from build123d import *

# Parameters (mm, degrees)
BOSS_EXTRUDE1_DEPTH      = 3
BOSS_EXTRUDE1_DEPTH_BACK = 4.55
SKETCH1_W                = 12
SKETCH1_H                = 10
SKETCH1_R                = 2.3
SKETCH1_H_2              = 28.075
SKETCH1_W_2              = 46.7
SKETCH5_W                = 12
SKETCH5_H                = 25.875
SKETCH5_H_2              = 10
SKETCH5_H_3              = 25.866
SKETCH5_W_2              = 46.7
CUT_EXTRUDE1_DEPTH       = 4.55
CUT_EXTRUDE2_DEPTH       = 87.014737759
CHAMFER1_SIZE            = 2
FILLET1_R                = 3
FILLET2_R                = 3


with BuildPart() as part:
    # Sketch1 → Boss-Extrude1 (new, two sides: drawn at the far end of the back side and taken through both)
    # profile 1 of 11: a face of its own
    with BuildSketch(Plane.XY.offset(-BOSS_EXTRUDE1_DEPTH_BACK)):
        with Locations((-38.872559152, 32.371494367)):
            Rectangle(SKETCH1_W, SKETCH1_H)
        with Locations((-38.872559152, 32.371494367)):
            Circle(SKETCH1_R, mode=Mode.SUBTRACT)
    # profile 2 of 11: a face of its own
    with BuildSketch(Plane.XY.offset(-BOSS_EXTRUDE1_DEPTH_BACK)):
        with Locations((-38.872559152, 13.333994367)):
            Rectangle(SKETCH1_W, SKETCH1_H_2)
    # profile 3 of 11: a face of its own
    with BuildSketch(Plane.XY.offset(-BOSS_EXTRUDE1_DEPTH_BACK)):
        with Locations((-38.872559152, -5.703505633)):
            Rectangle(SKETCH1_W, SKETCH1_H)
    # profile 4 of 11: a face of its own
    with BuildSketch(Plane.XY.offset(-BOSS_EXTRUDE1_DEPTH_BACK)):
        with Locations((-38.872559152, -24.741005633)):
            Rectangle(SKETCH1_W, SKETCH1_H_2)
    # profile 5 of 11: a face of its own
    with BuildSketch(Plane.XY.offset(-BOSS_EXTRUDE1_DEPTH_BACK)):
        with Locations((-38.872559152, -43.778505633)):
            Rectangle(SKETCH1_W, SKETCH1_H)
        with Locations((-38.872559152, -43.778505633)):
            Circle(SKETCH1_R, mode=Mode.SUBTRACT)
    # profile 6 of 11: a face of its own
    with BuildSketch(Plane.XY.offset(-BOSS_EXTRUDE1_DEPTH_BACK)):
        with Locations((19.827440848, -24.741005633)):
            Rectangle(SKETCH1_W, SKETCH1_H_2)
    # profile 7 of 11: a face of its own
    with BuildSketch(Plane.XY.offset(-BOSS_EXTRUDE1_DEPTH_BACK)):
        with Locations((19.827440848, -43.778505633)):
            Rectangle(SKETCH1_W, SKETCH1_H)
        with Locations((19.827440848, -43.778505633)):
            Circle(SKETCH1_R, mode=Mode.SUBTRACT)
    # profile 8 of 11: a face of its own
    with BuildSketch(Plane.XY.offset(-BOSS_EXTRUDE1_DEPTH_BACK)):
        with Locations((19.827440848, -5.703505633)):
            Rectangle(SKETCH1_W, SKETCH1_H)
    # profile 9 of 11: a face of its own
    with BuildSketch(Plane.XY.offset(-BOSS_EXTRUDE1_DEPTH_BACK)):
        with Locations((-9.522559152, -5.703505633)):
            Rectangle(SKETCH1_W_2, SKETCH1_H)
    # profile 10 of 11: a face of its own
    with BuildSketch(Plane.XY.offset(-BOSS_EXTRUDE1_DEPTH_BACK)):
        with Locations((19.827440848, 13.333994367)):
            Rectangle(SKETCH1_W, SKETCH1_H_2)
    # profile 11 of 11: a face of its own
    with BuildSketch(Plane.XY.offset(-BOSS_EXTRUDE1_DEPTH_BACK)):
        with Locations((19.827440848, 32.371494367)):
            Rectangle(SKETCH1_W, SKETCH1_H)
        with Locations((19.827440848, 32.371494367)):
            Circle(SKETCH1_R, mode=Mode.SUBTRACT)
    extrude(amount=BOSS_EXTRUDE1_DEPTH + BOSS_EXTRUDE1_DEPTH_BACK)

    # Sketch5 → Cut-Extrude1 (cut)
    with BuildSketch(Plane(origin=(0, 0, -4.55), x_dir=(-1, 0, 0), z_dir=(0, 0, -1))):
        with Locations((-19.827440848, 12.233994367)):
            Rectangle(SKETCH5_W, SKETCH5_H)
        with Locations((-19.827440848, -5.703505633)):
            Rectangle(SKETCH5_W, SKETCH5_H_2)
        with Locations((-19.827440848, -23.636505633)):
            Rectangle(SKETCH5_W, SKETCH5_H_3)
        with Locations((9.522559152, -5.703505633)):
            Rectangle(SKETCH5_W_2, SKETCH5_H_2)
        with Locations((38.872559152, -5.703505633)):
            Rectangle(SKETCH5_W, SKETCH5_H_2)
        with Locations((38.872559152, -23.636505633)):
            Rectangle(SKETCH5_W, SKETCH5_H_3)
        with Locations((38.872559152, 12.233994367)):
            Rectangle(SKETCH5_W, SKETCH5_H)
    extrude(amount=-CUT_EXTRUDE1_DEPTH, mode=Mode.SUBTRACT)

    # Sketch6 → Cut-Extrude2 (cut, through all)
    with BuildSketch(Plane.ZY.offset(44.872559152)):
        Polygon((-1.05, 28.569847873), (3, 25.171494367), (3, 37.371494367), (-1.05, 37.371494367), align=None)
        Polygon((-1.05, -48.778505633), (3, -48.778505633), (3, -36.578505633), (-1.05, -39.976859139), align=None)
    extrude(amount=-CUT_EXTRUDE2_DEPTH, mode=Mode.SUBTRACT)

    # Chamfer1
    chamfer1_edges = [part.edges().sort_by_distance(p)[0] for p in [
        (-32.872559152, -10.703505633, 1.5),
        (13.827440848, -10.703505633, 1.5),
        (13.827440848, -0.703505633, 1.5),
        (-32.872559152, -0.703505633, 1.5),
    ]]
    chamfer(chamfer1_edges, length=CHAMFER1_SIZE)

    # Fillet1
    fillet1_edges = [part.edges().sort_by_distance(p)[0] for p in [
        (13.827440848, 37.371494367, -2.8),
        (25.827440848, 37.371494367, -2.8),
        (25.827440848, -48.778505633, -2.8),
        (13.827440848, -48.778505633, -2.8),
        (-32.872559152, -48.778505633, -2.8),
        (-44.872559152, -48.778505633, -2.8),
        (-44.872559152, 37.371494367, -2.8),
        (-32.872559152, 37.371494367, -2.8),
    ]]
    fillet(fillet1_edges, radius=FILLET1_R)

    # Fillet2
    fillet2_edges = [part.edges().sort_by_distance(p)[0] for p in [
        (-38.872559152, -36.578505633, 3),
        (-38.872559152, 25.171494367, 3),
        (19.827440848, 25.171494367, 3),
        (19.827440848, -36.578505633, 3),
    ]]
    fillet(fillet2_edges, radius=FILLET2_R)


solid = part.part
Input: part model. Units: mm. Frame: model coordinates. A direction names the side the tool comes from. Give positions to 0.01 mm unless a question says otherwise; leave off trailing zeros. Loops run counter-clockwise (first coordinate to the right, second up) from the corner with the lowest first, then second, coordinate; pieces in that order, holes last. Notation, with made-up numbers: M 63.25,44 L 122.25,44 A21 cw 122.25,81 Z; hole C 46.5,-1 d6. An arc over 180 degrees is marked long. Use one line per item in the form item = value.
1. Line query: L1, parallel to X at y = -17, z = 1.75; L2, parallel to Z at x = 19, y = -28; L3, parallel to Y at x = 4, z = 1. Output: solid intervals per line, ascending.
Numbers:
L1 = -44.87 to -32.87, 13.83 to 25.83
L2 = 0 to 3
L3 = -10.7 to -0.7
2. Pull-direction query (Z, two-part tool) for faces 5 (the face through (21, 30, -4.55)), 6 (the face through (-39, -36.57, -2)), 7 (the face through (20, 35, -1.05)); classes: released by +Z, released by -Z, zero draft, split by the parting line, or undercut.
Numbers:
face_5 = released by -Z
face_6 = zero draft
face_7 = released by +Z
3. Section query D-D, the plane x = -12. Return the cut outline in (y, z).
Numbers:
outline = M -10.7,0 L -0.7,0 L -0.7,3 L -10.7,3 Z
4. Section query C-C, the plane x = 21. Return the cut outline in (y, z), and give its area (3 significant figures).
Numbers:
outline = M -48.78,-4.55 L -45.76,-4.55 L -45.76,-1.05 L -48.78,-1.05 Z; M -41.8,-4.55 L -36.57,-4.55 L -36.57,0 L 25.17,0 L 25.17,-4.55 L 30.39,-4.55 L 30.39,-1.05 L 28.57,-1.05 L 26.07,1.93 A3 ccw 23.77,3 L -35.18,3 A3 ccw -37.48,1.93 L -39.98,-1.05 L -41.8,-1.05 Z; M 34.35,-4.55 L 37.37,-4.55 L 37.37,-1.05 L 34.35,-1.05 Z
area = 256 mm²
5. Section query A-A, the plane z = -3. Return the cut outline in (x, y), and give its area (3 significant figures).
Numbers:
outline = M -44.87,-45.78 A3 ccw -41.87,-48.78 L -35.87,-48.78 A3 ccw -32.87,-45.78 L -32.87,-36.57 L -44.87,-36.57 Z; M -44.87,25.17 L -32.87,25.17 L -32.87,34.37 A3 ccw -35.87,37.37 L -41.87,37.37 A3 ccw -44.87,34.37 Z; M 13.83,-45.78 A3 ccw 16.83,-48.78 L 22.83,-48.78 A3 ccw 25.83,-45.78 L 25.83,-36.57 L 13.83,-36.57 Z; M 13.83,25.17 L 25.83,25.17 L 25.83,34.37 A3 ccw 22.83,37.37 L 16.83,37.37 A3 ccw 13.83,34.37 Z; hole C -38.87,-43.78 d4.6; hole C -38.87,32.37 d4.6; hole C 19.83,-43.78 d4.6; hole C 19.83,32.37 d4.6
area = 504 mm²
6. Reachability of faces 1 (the face through (-39, 25.171, -2)), 2 (the face through (12.813, -11.69, 1.479)), 3 (the face through (19.7, -46.3, -1.05)), 4 (the face through (-31.887, 0.31, 1.479)) from +Z, -Z, +X, -X, +Y, -Y: full face, straight path, thin tool, end or side. Return the list, or none.
Numbers:
face_1 = -Z, +X, -X
face_2 = +Z, -Z, -Y
face_3 = +Z, +X, -X, -Y
face_4 = +Z, -Z, +Y
7. First-contact query: pin 1 (1.5 mm diameter, centred on x = -13, z = 1, fed in from +Y); pin 2 (3.5 mm diameter, centred on x = 19.83, y = -43.78, fed in from +Z); pin 3 (2.5 mm diameter, centred on x = 21, y = 34, fed in from +Z); pin 4 (18.5 mm diameter, centred on x = -8, y = -19.5, fed in from -Z). Flat tips, straight axial feed; report the tip coordinate or a pass-through.
Numbers:
pin_1 = -0.7
pin_2 = through
pin_3 = -1.05
pin_4 = 0
8. Section query B-B, the plane y = -20.5. Return the cut outline in (x, z).
Numbers:
outline = M -44.87,0 L -32.87,0 L -32.87,3 L -44.87,3 Z; M 13.83,0 L 25.83,0 L 25.83,3 L 13.83,3 Z
